from build123d import *

# Parameters (mm, degrees)
F0_R     = 88.9
F1_DEPTH = 3.175
F2_R     = 25.146
F2_R_2   = 22.606
F3_DEPTH = 53.975
F4_DEPTH = 12.7
F5_DEPTH = 12.7


with BuildPart() as f1:
    # F0 (on Top) → F1 (new body)
    with BuildSketch(Plane.XY):
        Circle(F0_R)
    extrude(amount=F1_DEPTH)

    # F2 (on Top) → F3 (join)
    with BuildSketch(Plane.XY):
        with Locations((-34.0220481157, 41.3056388497)):
            Circle(F2_R)
        with Locations((-34.0220481157, 41.3056388497)):
            Circle(F2_R_2, mode=Mode.SUBTRACT)
        with Locations((32.6357856393, 41.5858998895)):
            Circle(F2_R)
        with Locations((32.6357856393, 41.5858998895)):
            Circle(F2_R_2, mode=Mode.SUBTRACT)
    extrude(amount=F3_DEPTH)

    # F4 (cut, symmetric): a face of the model
    f4_faces = [f1.faces().sort_by_distance(p)[0] for p in [
        (-34.0220481157, 41.3056388497, 3.175),
    ]]
    extrude(f4_faces, amount=F4_DEPTH, both=True, mode=Mode.SUBTRACT)

    # F5 (cut, symmetric): a face of the model
    f5_faces = [f1.faces().sort_by_distance(p)[0] for p in [
        (32.6357856393, 41.5858998895, 3.175),
    ]]
    extrude(f5_faces, amount=F5_DEPTH, both=True, mode=Mode.SUBTRACT)


solid = f1.part
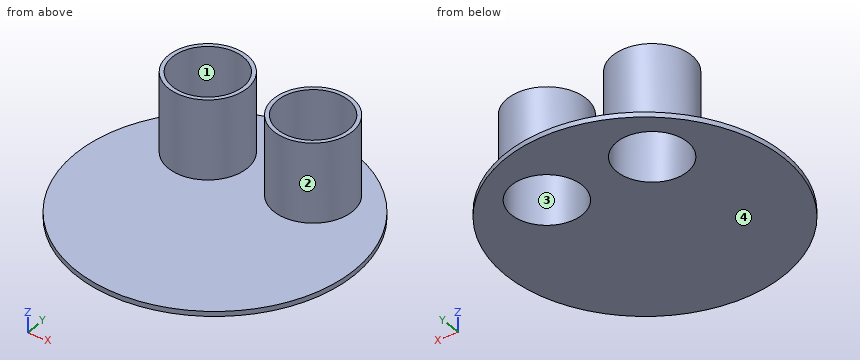
Input: part model. Units: mm. Frame: model coordinates. Face numbers are marked on the shaded views. A direction names the side the tool comes from. Coordinates: 2 decimals unless noted, no trailing zeros. Order: outer loops, then holes, each group sorted by start corner. A loop starts at its lowest first (then second) coordinate and runs counter-clockwise, first axis right, second up.
1. Ray query, line 1 along X through (y, z) = (38, 31.5); line 2 along Z through (x, y) = (-13, -71) (3 decimals); line 3 along Y through (x, z) = (13.5, 21). Return the intervals inside material, ascending.
Checked values:
line 1: x = -58.95 to -56.39, -11.66 to -9.09, 7.75 to 10.32, 54.96 to 57.52
line 2: z = 0 to 3.175
line 3: y = 25.27 to 29.55, 53.62 to 57.9
2. Cut plane B-B, the plane y = 0. Return loops of the section in (x, z) (3 decimals), plus the area to 3 significant figures.
Checked values:
outline: (-88.9, 0) - (88.9, 0) - (88.9, 3.175) - (-88.9, 3.175) - close
area: 565 mm2
3. Access query for the marked faces 1 and 2. Directions: +Z, -Z, +X, -X, +Y, -Y. A direction counts if a zero-diameter tool reaches every point of the face in a straight line with its end or side. Return the directions, or none.
Checked values:
face 1: +Z, -Z
face 2: +Z
4. Cut plane A-A, the plane z = 36.5. Return loops of the section in (x, y), plus the area to 3 significant figures.
Checked values:
outline: circle Ø50.29 at (-34.02, 41.31); circle Ø50.29 at (32.64, 41.59); hole circle Ø45.21 at (-34.02, 41.31); hole circle Ø45.21 at (32.64, 41.59)
area: 762 mm2
5. Draft query along X for the marked faces 3 and 4. Return one class per face: +X half, -X half, draft (parallel to the pull), parting line (faces both ways), or undercut.
Checked values:
face 3: undercut
face 4: draft
6. Contact query for flat-ended pins moving along their axis: P1, Ø10, axis at x = 36.5, y = -3, coming from the +Z side (3 decimals); P2, Ø10, axis at x = 38, z = 22.5, coming from the -Y side; P3, Ø3, axis at x = 60, z = 27.5, coming from the +Y side; P4, Ø6, axis at x = 29.5, z = 6, coming from the -Y side. Output: stop coordinate, or through.
Checked values:
P1: stops at z = 3.175
P2: stops at y = 16.44
P3: passes through
P4: stops at y = -84.21
